Study the drawing (mm; zero at the part's minimum x, y, z) and answer. A direction names the side the tool comes from. Coordinates: 2 decimals unless noted, no trailing zeros. Loops run counter-clockwise (first coordinate to the right, second up) from the corner with the lowest first, then second, coordinate; pieces in that order, holes last. Notation, with made-up numbers: (64, -7.75) - (119, -7.75) arc R15 cw to (119, 1.25) - close; hole circle Ø2 at (80, -25.75). An arc over 180 degrees is marked (long way). Use one line per item in the form item = value. Start each with the question number.
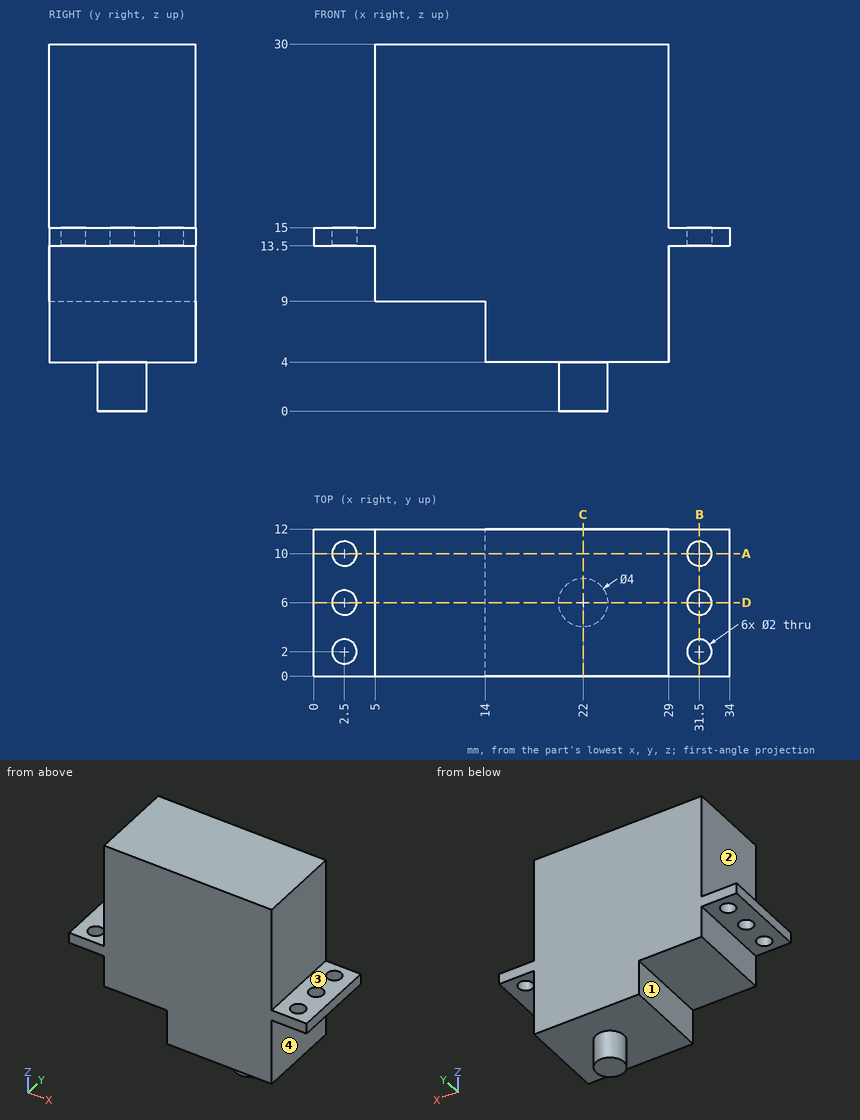
(1) Each of these flat-tipped pins is pushed along its axis until it touches: pin 1 Ø6 at (y, z) = (10, 5.5) entering from -X; pin 2 Ø3 at (x, y) = (31.5, 2) entering from -Z; pin 3 Ø3.5 at (y, z) = (8, 23.5) entering from +X. Where does it stop, or does it pass through?
(2) A cutting plane is placed at C-C (x = 22). Determine the outline of the cut face in (y, z), then the cut area to 3 significant figures.
(3) A cutting plane is placed at A-A (y = 10). Determine the outline of the cut face in (x, z).
(4) For the marked faces 1, 2, 3 and 4, determine the directions among +Z, -Z, +X, -X, +Y, -Y from which every point of the face is accessible in a straight line to the end or side of a thin tool.
(5) A cutting plane is placed at D-D (y = 6). Determine the outline of the cut face in (x, z), then the cut area to 3 significant figures.
(6) Find the intervals of material crossed by probe 1 along Y at (x, z) = (2.5, 14.35); probe 2 along Z at (x, y) = (25, 8); probe 3 along X at (y, z) = (11.75, 4.5), in increasing order. Write a range as from..to.
(7) A cutting plane is placed at B-B (x = 31.5). Determine the outline of the cut face in (y, z), then the cut area to 3 significant figures.
Evaluation:
q1.pin_1 = 14
q1.pin_2 = 13.5
q1.pin_3 = 29
q2.outline = (0, 4) - (4, 4) - (4, 0) - (8, 0) - (8, 4) - (12, 4) - (12, 30) - (0, 30) - close
q2.area = 328 mm^2
q3.outline = (0, 13.5) - (1.5, 13.5) - (1.5, 15) - (0, 15) - close; (3.5, 13.5) - (5, 13.5) - (5, 9) - (14, 9) - (14, 4) - (29, 4) - (29, 13.5) - (30.5, 13.5) - (30.5, 15) - (29, 15) - (29, 30) - (5, 30) - (5, 15) - (3.5, 15) - close; (32.5, 13.5) - (34, 13.5) - (34, 15) - (32.5, 15) - close
q4.face_1 = -Z, -X, +Y, -Y
q4.face_2 = +Z, -X, +Y, -Y
q4.face_3 = +Z, +X, +Y, -Y
q4.face_4 = -Z, +X, +Y, -Y
q5.outline = (0, 13.5) - (1.5, 13.5) - (1.5, 15) - (0, 15) - close; (3.5, 13.5) - (5, 13.5) - (5, 9) - (14, 9) - (14, 4) - (20, 4) - (20, 0) - (24, 0) - (24, 4) - (29, 4) - (29, 13.5) - (30.5, 13.5) - (30.5, 15) - (29, 15) - (29, 30) - (5, 30) - (5, 15) - (3.5, 15) - close; (32.5, 13.5) - (34, 13.5) - (34, 15) - (32.5, 15) - close
q5.area = 604 mm^2
q6.probe_1 = 0..1, 3..5, 7..9, 11..12
q6.probe_2 = 4..30
q6.probe_3 = 14..29
q7.outline = (0, 13.5) - (1, 13.5) - (1, 15) - (0, 15) - close; (3, 13.5) - (5, 13.5) - (5, 15) - (3, 15) - close; (7, 13.5) - (9, 13.5) - (9, 15) - (7, 15) - close; (11, 13.5) - (12, 13.5) - (12, 15) - (11, 15) - close
q7.area = 9.00 mm^2
